Read the model definition and answer for the solid it produces. Units are mm, in the model's axes. Face numbers are marked on the shaded views. A direction names the side the tool comes from. Coordinates: 2 decimals unless noted, no trailing zeros. Order: outer loops, then holes, each group sorted by start corner. A loop starts at its lowest first (then second) coordinate and runs counter-clockwise, first axis right, second up.
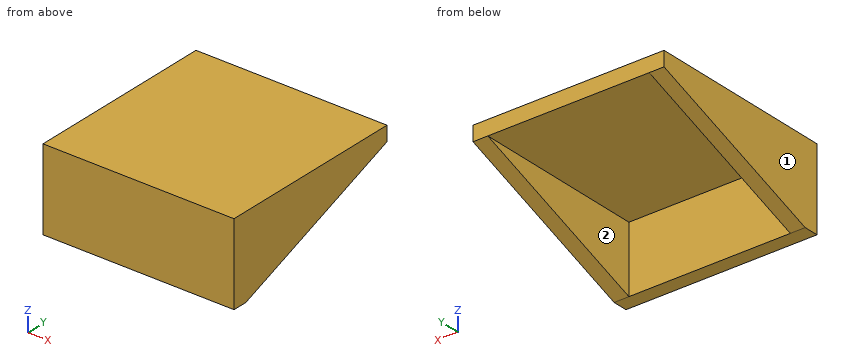
```python
from build123d import *

# Parameters (mm, degrees)
EXTRUDE_THIN1_DEPTH = 64.5
EXTRUDE1_DEPTH      = 10


with BuildPart() as part:
    # Sketch1 → Extrude-Thin1 (new body, symmetric)
    with BuildSketch(Plane(origin=(0, 0, 0), x_dir=(0, 0, -1), z_dir=(1, 0, 0))):
        Polygon((0, 129), (0, 0), (55, 0), (55, 10), (10, 10), (10, 129), align=None)
    extrude(amount=EXTRUDE_THIN1_DEPTH, both=True)

    # Sketch2 → Extrude1 (add)
    with BuildSketch(Plane(origin=(64.5, 0, 0), x_dir=(0, 0, -1), z_dir=(1, 0, 0))):
        Polygon((10, 129), (55, 10), (10, 10), align=None)
    extrude1 = extrude(amount=-EXTRUDE1_DEPTH)

    # Mirror1: Extrude1 across plane
    add(extrude1.mirror(Plane(origin=(0, 0, 0), x_dir=(0, 0, 1), z_dir=(1, 0, 0))))


solid = part.part
```
1) A cutting plane is placed at C-C, the plane y = 121.5. Determine the outline of the cut face in (x, z), and give its area (3 significant figures).
A:
outline: (-64.5, -12.84) - (-54.5, -12.84) - (-54.5, -10) - (54.5, -10) - (54.5, -12.84) - (64.5, -12.84) - (64.5, 0) - (-64.5, 0) - close
area: 1,350 mm2
2) A cutting plane is placed at B-B, the plane z = -39. Determine the outline of the cut face in (x, y), and give its area (3 significant figures).
A:
outline: (-64.5, 0) - (64.5, 0) - (64.5, 52.31) - (54.5, 52.31) - (54.5, 10) - (-54.5, 10) - (-54.5, 52.31) - (-64.5, 52.31) - close
area: 2,140 mm2
3) A cutting plane is placed at A-A, the plane x = 12. Determine the outline of the cut face in (y, z), and give its area (3 significant figures).
A:
outline: (0, -55) - (10, -55) - (10, -10) - (129, -10) - (129, 0) - (0, 0) - close
area: 1,740 mm2
4) Straight lines are drawn through the part: line 1 (X direction, y = 28.5, z = -42); line 2 (Y direction, x = -9.5, z = -35); line 3 (Z direction, x = 36.5, y = 110.5). For each, find the intervals that lie inside material, in ascending order.
A:
line 1: x = -64.5 to -54.5, 54.5 to 64.5
line 2: y = 0 to 10
line 3: z = -10 to 0
5) Flat-ended cylindrical pins translate along their axes: pin 1 Ø10 at (x, z) = (-12.5, -47.5) entering from +Y; pin 2 Ø1 at (x, y) = (6.5, 43.5) entering from -Z. Find the tip coordinate at first contact, or state that the pin passes through.
A:
pin 1: stops at y = 10
pin 2: stops at z = -10
6) Which of the six approach directions +Z, -Z, +X, -X, +Y, -Y give full straight-line access (tool end or side, diameter ignored) to the marked faces 1 and 2?
A:
face 1: +Z, -Z, -X, +Y, -Y
face 2: -Z, +Y
